Can you work these out from the drawing? Everything is in mm from the part's minimum corner. Round coordinates to 2 decimals unless told otherwise and drop trailing zeros. Order: outer loops, then holes, each group sorted by start corner. A loop starts at its lowest first (then second) coordinate and runs counter-clockwise, first axis right, second up. Notation, with made-up numbers: M 33,82.25 L 66,82.25 A20 cw 66,93.25 Z; hole C 22,-22.5 d5. An arc over 180 degrees is marked long. Answer as CSV lines item,"result". Start each with the question number.
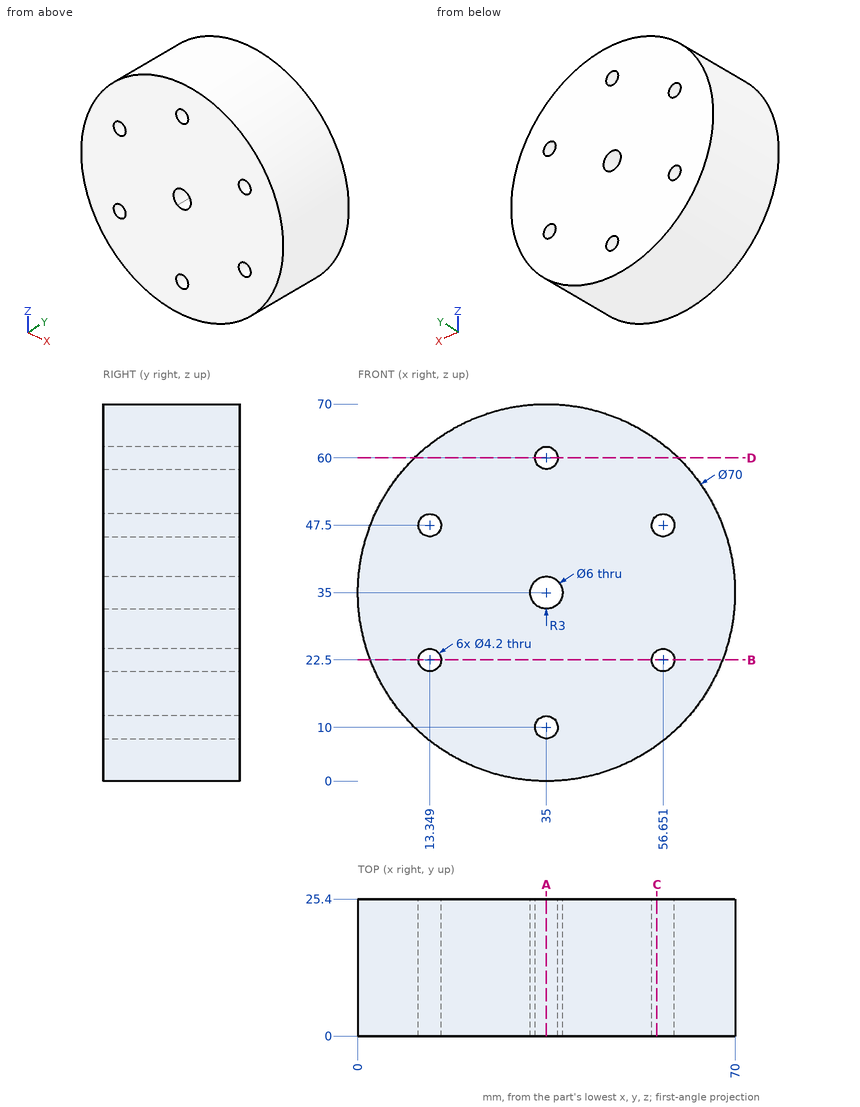
(1) I want a section at D-D on z = 60. Write out the boundary of the cut face in (x, y) (1 decimal).
(2) I'm going to push flat-ended pins straight in: P1, Ø6, axis at x = 49, y = 9, coming from the +Z side; P2, Ø6.5, axis at x = 13.35, z = 22.5, coming from the +Y side; P3, Ø12, axis at y = 15.5, z = 63, coming from the -X side; P4, Ø12, axis at y = 14, z = 20, coming from the +X side. Where does each tip first touch, or does it pass through?
(3) I want a section at C-C on x = 55.5. Write out the boundary of the cut face in (y, z), and give its area (3 significant figures).
(4) I want a section at B-B on z = 22.5. Write out the boundary of the cut face in (x, y), and give its area (3 significant figures).
(5) I want a section at A-A on x = 35. Write out the boundary of the cut face in (y, z).
(6) If I drill on line 1 along X through (y, z) = (19, 35); line 2 along X through (y, z) = (7, 22.5); line 3 along Z through (x, y) = (13, 20.5), over which ranges is the centre line in solid material (lowest first)?
From the geometry:
1,outline,"M 10.5,0 L 32.9,0 L 32.9,25.4 L 10.5,25.4 Z; M 37.1,0 L 59.5,0 L 59.5,25.4 L 37.1,25.4 Z"
2,P1,"z = 68.23"
2,P2,"y = 25.4"
2,P3,"x = 7.78"
2,P4,"x = 68.82"
3,outline,"M 0,6.63 L 25.4,6.63 L 25.4,20.74 L 0,20.74 Z; M 0,24.26 L 25.4,24.26 L 25.4,45.74 L 0,45.74 Z; M 0,49.26 L 25.4,49.26 L 25.4,63.37 L 0,63.37 Z"
3,area,"1,260 mm²"
4,outline,"M 2.31,0 L 11.25,0 L 11.25,25.4 L 2.31,25.4 Z; M 15.45,0 L 54.55,0 L 54.55,25.4 L 15.45,25.4 Z; M 58.75,0 L 67.69,0 L 67.69,25.4 L 58.75,25.4 Z"
4,area,"1,450 mm²"
5,outline,"M 0,0 L 25.4,0 L 25.4,7.9 L 0,7.9 Z; M 0,12.1 L 25.4,12.1 L 25.4,32 L 0,32 Z; M 0,38 L 25.4,38 L 25.4,57.9 L 0,57.9 Z; M 0,62.1 L 25.4,62.1 L 25.4,70 L 0,70 Z"
6,line 1,"0 to 32, 38 to 70"
6,line 2,"2.31 to 11.25, 15.45 to 54.55, 58.75 to 67.69"
6,line 3,"7.78 to 20.43, 24.57 to 45.43, 49.57 to 62.22"
